For this review, use the dimensioned drawing (mm, ordinates from the lowest corner) and the shaded views. A direction names the side the tool comes from. Coordinates: 2 decimals unless noted, no trailing zeros. Loops run counter-clockwise (first coordinate to the right, second up) from the corner with the lowest first, then second, coordinate; pieces in that order, holes last. Notation, with made-up numbers: (-13, 68.25) -> (-4, 68.25) arc R22 cw to (-4, 86.25) -> close; hole circle Ø6 at (64, -15). An arc over 180 degrees is marked (long way). Use one line per item in the form item = value. Start each with the question number.
1. Consider section A-A (z = 6.75). State the section outline as (x, y) points.
2. Wall thickness on line 1 (Y direction, x = 18, z = 6); line 2 (X direction, y = 3.8, z = 6) (1 decimal); line 3 (X direction, y = 2.35, z = 1.75) (1 decimal): over which ranges is each line inside the solid? List them lowest first. Write a range as from..to.
3. For pin 1 (1 mm diameter, centred on y = 4.5, z = 6.5, fed in from -X), flat-tipped, find the tip position at first contact; note if it passes through.
4. Consider section D-D (z = 3.5). State the section outline as (x, y) points.
5. Machinability: for the marked faces 5 and 6, which of the approach directions +Z, -Z, +X, -X, +Y, -Y give a long, thin tool a straight path to every point of the face, cutting with its end or side? Answer none if there is none.
6. Consider section B-B (y = 3). State the section outline as (x, z) points.
7. The part is to be moulded in two halves that separate along X. For the marked faces 1, 2, 3 and 4, say which applies: released by +X, released by -X, zero draft, split by the parting line, or undercut.
8. Consider section C-C (x = 17.5). State the section outline as (y, z) points, then the cut area to 3 significant figures.
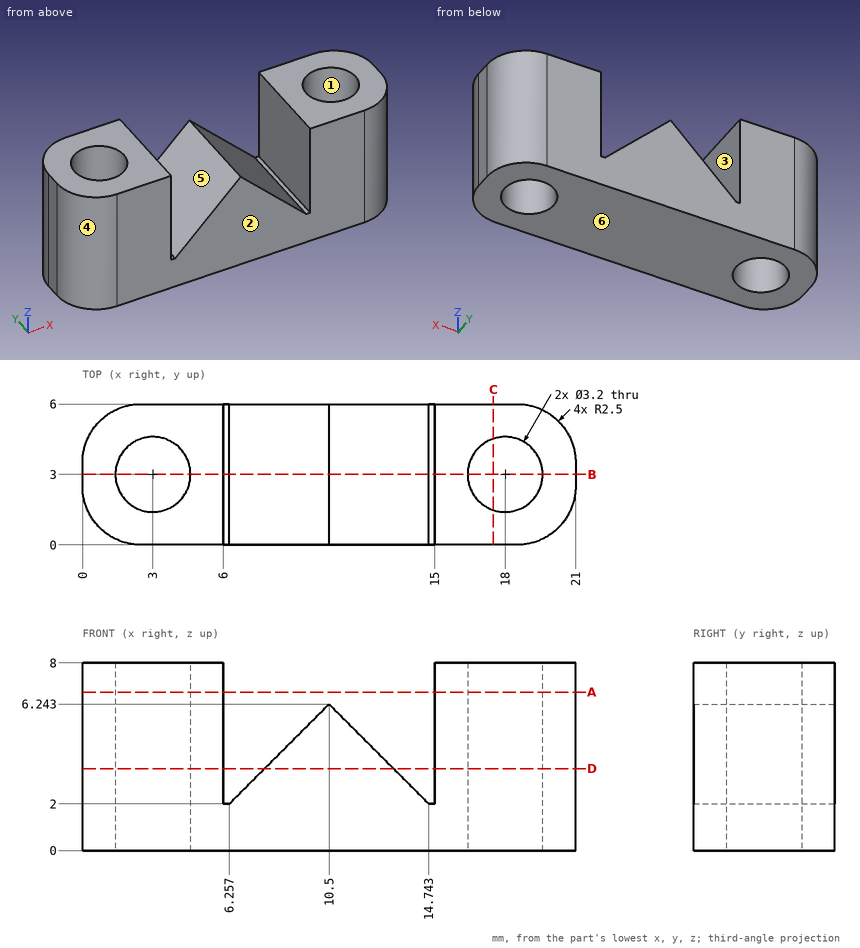
Geometry check:
q1.outline = (0, 2.5) arc R2.5 ccw to (2.5, 0) -> (6, 0) -> (6, 6) -> (2.5, 6) arc R2.5 ccw to (0, 3.5) -> close; (15, 0) -> (18.5, 0) arc R2.5 ccw to (21, 2.5) -> (21, 3.5) arc R2.5 ccw to (18.5, 6) -> (15, 6) -> close; hole circle Ø3.2 at (3, 3); hole circle Ø3.2 at (18, 3)
q2.line_1 = 0..1.4, 4.6..6
q2.line_2 = 0..1.6, 4.4..6, 10.3..10.7, 15..16.6, 19.4..21
q2.line_3 = 0..1.5, 4.5..16.5, 19.5..21
q3.pin_1 = 0.05
q4.outline = (0, 2.5) arc R2.5 ccw to (2.5, 0) -> (6, 0) -> (6, 6) -> (2.5, 6) arc R2.5 ccw to (0, 3.5) -> close; (7.76, 0) -> (13.24, 0) -> (13.24, 6) -> (7.76, 6) -> close; (15, 0) -> (18.5, 0) arc R2.5 ccw to (21, 2.5) -> (21, 3.5) arc R2.5 ccw to (18.5, 6) -> (15, 6) -> close; hole circle Ø3.2 at (3, 3); hole circle Ø3.2 at (18, 3)
q5.face_5 = +Z, +Y, -Y
q5.face_6 = -Z, +X, -X, +Y, -Y
q6.outline = (0, 0) -> (1.4, 0) -> (1.4, 8) -> (0, 8) -> close; (4.6, 0) -> (16.4, 0) -> (16.4, 8) -> (15, 8) -> (15, 2) -> (14.74, 2) -> (10.5, 6.24) -> (6.26, 2) -> (6, 2) -> (6, 8) -> (4.6, 8) -> close; (19.6, 0) -> (21, 0) -> (21, 8) -> (19.6, 8) -> close
q7.face_1 = undercut
q7.face_2 = zero draft
q7.face_3 = undercut
q7.face_4 = released by -X
q8.outline = (0, 0) -> (1.48, 0) -> (1.48, 8) -> (0, 8) -> close; (4.52, 0) -> (6, 0) -> (6, 8) -> (4.52, 8) -> close
q8.area = 23.7 mm²
